Geometry: final body of the model. Coordinates: model frame, mm. A direction names the side the tool comes from. Give positions to 0.01 mm unless a question says otherwise; leave off trailing zeros. Write each loop counter-clockwise with the first axis right and the second up, starting at its lowest first coordinate (ties: lowest second). Pieces come first, ordered by that corner, then holes. Notation, with made-up numbers: M -15.5,-18 L 15.5,-18 A4 cw 15.5,-13 Z; hole C -30.75,-13.75 d10. An arc over 180 degrees is marked long. Use a Markdown table: item, result. Add a question column.
1) Section D-D on y = -34. Return the cut outline in (x, z), then the cut area to 3 significant figures.
2) Section A-A on z = -2. Return the cut outline in (x, y), then the cut area to 3 significant figures.
3) Pin query (flat end, axial travel): pin 1 (10 mm diameter, centred on x = -7.5, y = 26.5, fed in from -Z); pin 2 (3 mm diameter, centred on y = 41, z = 1.5, fed in from -X) (3 decimals). Return the tip coordinate at first contact, or that it passes through.
4) Draft query along X for faces 1 (the flat face through (-11.815, -35, 2)), 2 (the cylindrical face through (-6.397, -40.046, -2.465)), 3 (the flat face through (-8, 16, -5)). Return one class per face: +X half, -X half, draft (parallel to the pull), parting line (faces both ways), or undercut.
5) Section C-C on z = 1.75. Return the cut outline in (x, y), then the cut area to 3 significant figures.
6) Set-up query: faces 4 (the cylindrical face through (-7.21, 57.615, -2.465)), 5 (the flat face through (-2, -42.826, 2)), 6 (the flat face through (-4, 43.174, 2)). Return all of +Z, -Z, +X, -X, +Y, -Y with unobstructed straight access to the full face (end or side cutting, diameter ignored); none if empty.
7) Section B-B on x = 0. Return the cut outline in (y, z), then the cut area to 3 significant figures.
8) Line query: line 1 (Y direction, x = -7, z = 2.25); line 2 (X direction, y = 1, z = -1.25); line 3 (Z direction, x = 3.75, y = 49). Output: solid intervals per line, ascending.
```python
from build123d import *

# Parameters (mm, degrees)
EXTRUDE_1_DEPTH     = 3.5
SKETCH_2_W          = 60
SKETCH_2_H          = 102
CUT_EXTRUDE_1_DEPTH = 3.5
SKETCH_7_W          = 3.5
SKETCH_7_H          = 16
EXTRUDE_3_DEPTH     = 15
SKETCH_6_R          = 2.5
SKETCH_6_R_2        = 1.25
EXTRUDE_2_DEPTH     = 5


with BuildPart() as part:
    # 草图1 → 凸台-拉伸1 (new body)
    with BuildSketch(Plane.XY):
        Polygon((68.184988255, 39.174258776), (68.184988255, -22.825741224), (68.184988255, -42.825741224), (3.184988255, -42.825741224), (3.184988255, -22.825741224), (-11.815011745, -22.825741224), (-11.815011745, 39.174258776), (3.184988255, 39.174258776), (3.184988255, 59.174258776), (68.184988255, 59.174258776), align=None)
    extrude(amount=EXTRUDE_1_DEPTH)

    # 草图2 → 切除-拉伸1 (cut)
    with BuildSketch(Plane.XY.offset(3.5)):
        with Locations((38.184988255, 8.174258776)):
            Rectangle(SKETCH_2_W, SKETCH_2_H)
    extrude(amount=-CUT_EXTRUDE_1_DEPTH, mode=Mode.SUBTRACT)

    # 草图7 → 凸台-拉伸3 (add)
    with BuildSketch(Plane.ZY.offset(-3.184988255)):
        with Locations((1.75, 51.174258776)):
            Rectangle(SKETCH_7_W, SKETCH_7_H)
        with Locations((1.75, -34.825741224)):
            Rectangle(SKETCH_7_W, SKETCH_7_H)
    extrude(amount=EXTRUDE_3_DEPTH)

    # 草图6 → 凸台-拉伸2 (add)
    # profile 1 of 4: a face of its own
    with BuildSketch(Plane(origin=(0, 0, 0), x_dir=(-1, 0, 0), z_dir=(0, 0, -1))):
        with Locations(Location((6.668106828, -38.825741224, 0), (0, 0, 180))):
            Circle(SKETCH_6_R)
        with Locations((6.668106828, -38.825741224)):
            Circle(SKETCH_6_R_2, mode=Mode.SUBTRACT)
    # profile 2 of 4: a face of its own
    with BuildSketch(Plane(origin=(0, 0, 0), x_dir=(-1, 0, 0), z_dir=(0, 0, -1))):
        with Locations(Location((6.668106828, 1.174258776, 0), (0, 0, 180))):
            Circle(SKETCH_6_R)
        with Locations((6.668106828, 1.174258776)):
            Circle(SKETCH_6_R_2, mode=Mode.SUBTRACT)
    # profile 3 of 4: a face of its own
    with BuildSketch(Plane(origin=(0, 0, 0), x_dir=(-1, 0, 0), z_dir=(0, 0, -1))):
        with Locations(Location((6.668106828, 15.174258776, 0), (0, 0, 180))):
            Circle(SKETCH_6_R)
        with Locations((6.668106828, 15.174258776)):
            Circle(SKETCH_6_R_2, mode=Mode.SUBTRACT)
    # profile 4 of 4: a face of its own
    with BuildSketch(Plane(origin=(0, 0, 0), x_dir=(-1, 0, 0), z_dir=(0, 0, -1))):
        with Locations(Location((6.668106828, 55.174258776, 0), (0, 0, 180))):
            Circle(SKETCH_6_R)
        with Locations((6.668106828, 55.174258776)):
            Circle(SKETCH_6_R_2, mode=Mode.SUBTRACT)
    extrude(amount=EXTRUDE_2_DEPTH)


solid = part.part
```
Found:
| question | item | result |
|---|---|---|
| 1 | outline | M -11.82,0 L 8.18,0 L 8.18,3.5 L -11.82,3.5 Z |
| 1 | area | 70.0 mm² |
| 2 | outline | C -6.67,-38.83 d5; C -6.67,1.17 d5; C -6.67,15.17 d5; C -6.67,55.17 d5; hole C -6.67,-38.83 d2.5; hole C -6.67,1.17 d2.5; hole C -6.67,15.17 d2.5; hole C -6.67,55.17 d2.5 |
| 2 | area | 58.9 mm² |
| 3 | pin 1 | z = 0 |
| 3 | pin 2 | x = 3.185 |
| 4 | face 1 | -X half |
| 4 | face 2 | undercut |
| 4 | face 3 | draft |
| 5 | outline | M -11.82,-42.83 L 8.18,-42.83 L 8.18,59.17 L -11.82,59.17 L -11.82,43.17 L 3.18,43.17 L 3.18,39.17 L -11.82,39.17 L -11.82,-22.83 L 3.18,-22.83 L 3.18,-26.83 L -11.82,-26.83 Z |
| 5 | area | 1,920 mm² |
| 6 | face 4 | -Z |
| 6 | face 5 | +Z, -Z, +X, -X, -Y |
| 6 | face 6 | +Z, -Z, -X |
| 7 | outline | M -42.83,0 L -26.83,0 L -26.83,3.5 L -42.83,3.5 Z; M -22.83,0 L 39.17,0 L 39.17,3.5 L -22.83,3.5 Z; M 43.17,0 L 59.17,0 L 59.17,3.5 L 43.17,3.5 Z |
| 7 | area | 329 mm² |
| 8 | line 1 | -42.83 to -26.83, -22.83 to 39.17, 43.17 to 59.17 |
| 8 | line 2 | -9.16 to -7.91, -5.43 to -4.17 |
| 8 | line 3 | 0 to 3.5 |
